Geometry check sheet. Reference: the model listing, model coordinates, mm. A direction names the side the tool comes from. Give positions to 0.01 mm unless a question says otherwise; leave off trailing zeros. Order: outer loops, then holes, each group sorted by start corner. A loop starts at its lowest first (then second) coordinate and runs counter-clockwise, first axis right, second up.
from build123d import *

# Parameters (mm, degrees)
SKETCH1_W           = 40
SKETCH1_H           = 40
BOSS_EXTRUDE1_DEPTH = 30
SKETCH2_W           = 20
SKETCH2_H           = 20
CUT_EXTRUDE1_DEPTH  = 20
SKETCH5_R           = 1.8
CUT_EXTRUDE6_DEPTH  = 20
SKETCH25_W          = 2
SKETCH25_H          = 10
BOSS_EXTRUDE2_DEPTH = 10
SKETCH26_W          = 2
SKETCH26_H          = 10
BOSS_EXTRUDE3_DEPTH = 10
SKETCH27_R          = 1.5
CUT_EXTRUDE7_DEPTH  = 10
CUT_EXTRUDE8_DEPTH  = 10
CUT_EXTRUDE9_DEPTH  = 10
SKETCH30_R          = 3
CUT_EXTRUDE10_DEPTH = 5


with BuildPart() as part:
    # Sketch1 → Boss-Extrude1 (new body)
    with BuildSketch(Plane.XY):
        with Locations((-5.074257426, 5)):
            Rectangle(SKETCH1_W, SKETCH1_H)
    extrude(amount=BOSS_EXTRUDE1_DEPTH)

    # Sketch2 → Cut-Extrude1 (cut)
    with BuildSketch(Plane(origin=(0, 0, 0), x_dir=(-1, 0, 0), z_dir=(0, 0, -1))):
        with Locations((5.074257426, 15)):
            Rectangle(SKETCH2_W, SKETCH2_H)
    extrude(amount=-CUT_EXTRUDE1_DEPTH, mode=Mode.SUBTRACT)

    # Sketch5 → Cut-Extrude6 (cut)
    with BuildSketch(Plane(origin=(0, 5, 0), x_dir=(1, 0, 0), z_dir=(0, 1, 0))):
        with Locations(Location((-5.074257426, -10, 0), (0, 0, 270))):
            Circle(SKETCH5_R)
    extrude(amount=-CUT_EXTRUDE6_DEPTH, mode=Mode.SUBTRACT)

    # Sketch24 → Cut-Revolve1 (revolve, cut)
    with BuildSketch(Plane.XY.offset(10), mode=Mode.PRIVATE) as cut_revolve1_sk:
        Polygon((-3.274257426, -5), (-5.074257426, -5), (-5.074257426, 5), (4.925742574, 5), align=None)
    revolve(cut_revolve1_sk.sketch.rotate(Axis((-5.074257426, 5, 10), (0, -1, 0)), 90), axis=Axis((-5.074257426, 5, 10), (0, -1, 0)), mode=Mode.SUBTRACT)

    # Sketch25 → Boss-Extrude2 (add)
    with BuildSketch(Plane.ZY.offset(25.074257426)):
        with Locations((1, -10)):
            Rectangle(SKETCH25_W, SKETCH25_H)
    extrude(amount=BOSS_EXTRUDE2_DEPTH)

    # Sketch26 → Boss-Extrude3 (add)
    with BuildSketch(Plane(origin=(14.925742574, 0, 0), x_dir=(0, 0, -1), z_dir=(1, 0, 0))):
        with Locations((-1, -10)):
            Rectangle(SKETCH26_W, SKETCH26_H)
    extrude(amount=BOSS_EXTRUDE3_DEPTH)

    # Sketch27 → Cut-Extrude7 (cut)
    with BuildSketch(Plane(origin=(0, 0, 0), x_dir=(-1, 0, 0), z_dir=(0, 0, -1))):
        with Locations((-19.925742574, -10)):
            Circle(SKETCH27_R)
        with Locations((30.074257426, -10)):
            Circle(SKETCH27_R)
    extrude(amount=-CUT_EXTRUDE7_DEPTH, mode=Mode.SUBTRACT)

    # Sketch28 → Cut-Extrude8 (cut)
    with BuildSketch(Plane(origin=(14.925742574, 0, 0), x_dir=(0, 0, -1), z_dir=(1, 0, 0))):
        Polygon((-15, -10), (-15, -15), (-5, -15), (-5, -10), (-2, -10), (-2, -5), (-18, -5), (-18, -10), align=None)
    extrude(amount=-CUT_EXTRUDE8_DEPTH, mode=Mode.SUBTRACT)

    # Sketch29 → Cut-Extrude9 (cut)
    with BuildSketch(Plane.ZY.offset(25.074257426)):
        Polygon((5, -15), (15, -15), (15, -10), (18, -10), (18, -5), (2, -5), (2, -10), (5, -10), align=None)
    extrude(amount=-CUT_EXTRUDE9_DEPTH, mode=Mode.SUBTRACT)

    # Sketch30 → Cut-Extrude10 (cut)
    with BuildSketch(Plane.XZ.offset(15)):
        with Locations(Location((-5.074257426, 10, 0), (0, 0, 270))):
            Circle(SKETCH30_R)
    extrude(amount=-CUT_EXTRUDE10_DEPTH, mode=Mode.SUBTRACT)


solid = part.part
Item 1: Set-up check for faces 1 (the flat face through (10, -5, 10)), 2 (the flat face through (10, -12, 15)), 3 (the flat face through (-20, -10, 3)), 4 (the flat face through (-15.074, 15, 10)), 5 (the flat face through (-30, -5, 1)): record each of +Z, -Z, +X, -X, +Y, -Y from which the full face is reachable in a straight line by a thin tool's end or side.
Reported:
face 1: +X
face 2: +X, -Y
face 3: -X
face 4: -Z, +Y
face 5: +Z, -Z, -X, +Y
Item 2: Sectioned sample at B-B (x = -29.5). Enter the section's corners in (y, z).
Reported:
outline: (-15, 0) - (-11.39, 0) - (-11.39, 2) - (-15, 2) - close; (-8.61, 0) - (-5, 0) - (-5, 2) - (-8.61, 2) - close
Item 3: Gauge pin test, flat ends, axial feed: pin 1 (6 mm diameter, centred on x = -11.5, y = 19.5, fed in from -Z); pin 2 (5 mm diameter, centred on y = 6, z = 22, fed in from +X); pin 3 (10 mm diameter, centred on x = -6, z = 11, fed in from +Y). Record the tip position at first contact, or that the pin passes through.
Reported:
pin 1: stops at z = 20
pin 2: stops at x = 14.93
pin 3: stops at y = 0.56
Item 4: Sectioned sample at C-C (x = 8). Enter the section's corners in (y, z).
Reported:
outline: (-15, 0) - (25, 0) - (25, 30) - (-15, 30) - (-15, 15) - (-10, 15) - (-10, 18) - (-5, 18) - (-5, 2) - (-10, 2) - (-10, 5) - (-15, 5) - close
Item 5: Scan lines: L1, parallel to X at y = 19.5, z = 11.5; L2, parallel to X at y = -8.4, z = 10; L3, parallel to Z at x = -21.5, y = -11.5. Record each from-to range of solid material in increasing order.
Reported:
L1: x = -25.07 to -15.07, 4.93 to 14.93
L2: x = -15.07 to -6.87, -3.27 to 4.93
L3: z = 0 to 5, 15 to 30
Item 6: Draft check along Z on faces 6 (the flat face through (4.926, 15, 10)), 7 (the flat face through (10, -7, 18)). Enter one of: released by +Z, released by -Z, zero draft, split by the parting line, or undercut.
Reported:
face 6: zero draft
face 7: undercut
Item 7: Sectioned sample at A-A (y = 1.5). Enter the section's corners in (x, z), and give its area (3 significant figures).
Reported:
outline: (-25.07, 0) - (14.93, 0) - (14.93, 30) - (-25.07, 30) - close; hole circle Ø14.26 at (-5.07, 10)
area: 1,040 mm2
Item 8: Sectioned sample at D-D (y = 6). Enter the section's corners in (x, z), and give its area (3 significant figures).
Reported:
outline: (-25.07, 0) - (-15.07, 0) - (-15.07, 20) - (4.93, 20) - (4.93, 0) - (14.93, 0) - (14.93, 30) - (-25.07, 30) - close
area: 800 mm2
